Could you check a few things on this model? Use its own coordinates, in mm. A direction names the side the tool comes from. Give positions to 0.01 mm unless a question says otherwise; leave off trailing zeros. Loops run counter-clockwise (first coordinate to the right, second up) from the corner with the lowest first, then second, coordinate; pieces in that order, holes last. Notation, with made-up numbers: (36, 51.25) - (77, 51.25) arc R22 cw to (77, 57.25) - close; hole circle Ø2 at (58.5, 76). An arc over 180 degrees is marked (long way). Use CSV: the item, a comma, the result in double quotes.
from build123d import *

# Parameters (mm, degrees)
BOSS_EXTRUDE1_DEPTH       = 2
BOSS_EXTRUDE2_DEPTH       = 21.5
FILLET1_R                 = 2
FILLET2_R                 = 2
BOSS_EXTRUDE3_START       = -22
BOSS_EXTRUDE3_OUTLINE_R   = 1.498302823
BOSS_EXTRUDE3_OUTLINE_R_2 = 1.5
BOSS_EXTRUDE3_DEPTH       = 22
FILLET3_R                 = 2


with BuildPart() as part:
    # Sketch3 → Boss-Extrude1 (new body)
    with BuildSketch(Plane.XY):
        Polygon((-15.640963985, -84.058941087), (4.526340861, -63.891636241), (4.526340861, -11.788708514), (100.581340861, -11.788708514), (100.581340861, -63.896636241), (120.743645706, -84.058941087), (120.743645706, -106.958318205), (104.551340861, -106.958318205), (-15.640963985, -106.958318205), (-15.640963985, -90.76601336), align=None)
    extrude(amount=-BOSS_EXTRUDE1_DEPTH)

    # Sketch3<3> → Boss-Extrude2 (add)
    with BuildSketch(Plane.XY):
        Polygon((-15.640963985, -90.76601336), (-15.640963985, -84.058941087), (4.526340861, -63.891636241), (4.526340861, -11.788708514), (100.581340861, -11.788708514), (100.581340861, -63.896636241), (120.743645706, -84.058941087), (120.743645706, -106.958318205), (104.551340861, -106.958318205), (-15.640963985, -106.958318205), align=None)
        Polygon((-13.840963985, -90.76601336), (-13.840963985, -105.158318205), (104.551340861, -105.158318205), (118.943645706, -105.158318205), (118.943645706, -84.804525499), (98.781340861, -64.642220653), (98.781340861, -13.588708514), (6.326340861, -13.588708514), (6.326340861, -64.637220653), (-13.840963985, -84.804525499), align=None, mode=Mode.SUBTRACT)
    extrude(amount=BOSS_EXTRUDE2_DEPTH)

    # Fillet1
    fillet1_edges = [part.edges().sort_by_distance(p)[0] for p in [
        (-15.640963985, -84.058941087, 9.75),
        (4.526340861, -63.891636241, 9.75),
        (4.526340861, -11.788708514, 9.75),
        (100.581340861, -11.788708514, 9.75),
        (100.581340861, -63.896636241, 9.75),
        (120.743645706, -84.058941087, 9.75),
        (120.743645706, -106.958318205, 9.75),
        (-15.640963985, -106.958318205, 9.75),
        (-13.840963985, -105.158318205, 10.75),
        (-13.840963985, -84.804525499, 10.75),
        (6.326340861, -64.637220653, 10.75),
        (6.326340861, -13.588708514, 10.75),
        (98.781340861, -13.588708514, 10.75),
        (98.781340861, -64.642220653, 10.75),
        (118.943645706, -105.158318205, 10.75),
    ]]
    fillet(fillet1_edges, radius=FILLET1_R)

    # Fillet2
    fillet2_edges = [part.edges().sort_by_distance(p)[0] for p in [
        (118.943645706, -84.804525499, 10.75),
    ]]
    fillet(fillet2_edges, radius=FILLET2_R)

    # Boss-Extrude3: read off the stored shape, not the designer's step
    # Boss-Extrude3 outline → Boss-Extrude3 (add)
    with BuildSketch(Plane.XY.offset(21.5).offset(BOSS_EXTRUDE3_START)):
        with BuildLine():
            ThreePointArc((101.167127298, -64.482422679), (100.733581796, -63.833575981), (100.581340861, -63.068209116))
            Line((100.581340861, -63.068209116), (100.581340861, -13.788708514))
            ThreePointArc((100.581340861, -13.788708514), (99.995554423, -12.374494952), (98.581340861, -11.788708514))
            Line((98.581340861, -11.788708514), (6.526340861, -11.788708514))
            ThreePointArc((6.526340861, -11.788708514), (5.112127298, -12.374494952), (4.526340861, -13.788708514))
            Line((4.526340861, -13.788708514), (4.526340861, -63.063209116))
            ThreePointArc((4.526340861, -63.063209116), (4.374099926, -63.828575981), (3.940554423, -64.477422679))
            Line((3.940554423, -64.477422679), (-15.055177547, -83.473154649))
            ThreePointArc((-15.055177547, -83.473154649), (-15.48872305, -84.122001347), (-15.640963985, -84.887368211))
            Line((-15.640963985, -84.887368211), (-15.640963985, -104.958318205))
            ThreePointArc((-15.640963985, -104.958318205), (-15.055177547, -106.372531767), (-13.640963985, -106.958318205))
            Line((-13.640963985, -106.958318205), (118.743645706, -106.958318205))
            ThreePointArc((118.743645706, -106.958318205), (120.157859269, -106.372531767), (120.743645706, -104.958318205))
            Line((120.743645706, -104.958318205), (120.743645706, -84.887368211))
            ThreePointArc((120.743645706, -84.887368211), (120.591404771, -84.122001347), (120.157859269, -83.473154649))
            Line((120.157859269, -83.473154649), (101.167127298, -64.482422679))
        make_face()
        with Locations((-12.195717461, -103.513071681)):
            Circle(BOSS_EXTRUDE3_OUTLINE_R, mode=Mode.SUBTRACT)
        with Locations((-1.913886606, -74.998768464)):
            Circle(BOSS_EXTRUDE3_OUTLINE_R_2, mode=Mode.SUBTRACT)
        with Locations((52.551340861, -103.658318205)):
            Circle(BOSS_EXTRUDE3_OUTLINE_R_2, mode=Mode.SUBTRACT)
        with Locations((117.297199097, -103.511871596)):
            Circle(BOSS_EXTRUDE3_OUTLINE_R_2, mode=Mode.SUBTRACT)
        with Locations((107.016568327, -74.998768464)):
            Circle(BOSS_EXTRUDE3_OUTLINE_R_2, mode=Mode.SUBTRACT)
        with BuildLine():
            ThreePointArc((-13.840963985, -85.632952624), (-13.68872305, -84.867585759), (-13.255177547, -84.218739061))
            Line((-13.255177547, -84.218739061), (-4.688095726, -75.651657241))
            ThreePointArc((-4.688095726, -75.651657241), (0.101367721, -77.01402279), (-1.260997829, -72.224559343))
            Line((-1.260997829, -72.224559343), (5.740554423, -65.223007091))
            ThreePointArc((5.740554423, -65.223007091), (6.174099926, -64.574160393), (6.326340861, -63.808793529))
            Line((6.326340861, -63.808793529), (6.326340861, -17.561464123))
            ThreePointArc((6.326340861, -17.561464123), (9.988041797, -17.25040945), (10.29909647, -13.588708514))
            Line((10.29909647, -13.588708514), (50.130516698, -13.588708514))
            ThreePointArc((50.130516698, -13.588708514), (52.553840861, -17.938708514), (54.977165024, -13.588708514))
            Line((54.977165024, -13.588708514), (94.808585252, -13.588708514))
            ThreePointArc((94.808585252, -13.588708514), (95.119639925, -17.25040945), (98.781340861, -17.561464123))
            Line((98.781340861, -17.561464123), (98.781340861, -63.813793529))
            ThreePointArc((98.781340861, -63.813793529), (98.933581796, -64.579160393), (99.367127298, -65.228007091))
            Line((99.367127298, -65.228007091), (106.36367955, -72.224559343))
            ThreePointArc((106.36367955, -72.224559343), (105.001314001, -77.01402279), (109.790777448, -75.651657241))
            Line((109.790777448, -75.651657241), (118.357859269, -84.218739061))
            ThreePointArc((118.357859269, -84.218739061), (118.791404771, -84.867585759), (118.943645706, -85.632952624))
            Line((118.943645706, -85.632952624), (118.943645706, -101.185562596))
            ThreePointArc((118.943645706, -101.185562596), (115.28194477, -101.496617269), (114.970890097, -105.158318205))
            Line((114.970890097, -105.158318205), (54.974665024, -105.158318205))
            ThreePointArc((54.974665024, -105.158318205), (52.551340861, -100.808318205), (50.128016698, -105.158318205))
            Line((50.128016698, -105.158318205), (-9.870638356, -105.158318205))
            ThreePointArc((-9.870638356, -105.158318205), (-10.18166322, -101.49901744), (-13.840963985, -101.187992576))
            Line((-13.840963985, -101.187992576), (-13.840963985, -85.632952624))
        make_face(mode=Mode.SUBTRACT)
        with Locations((7.97278747, -15.235155124)):
            Circle(BOSS_EXTRUDE3_OUTLINE_R_2, mode=Mode.SUBTRACT)
        with Locations((52.553840861, -15.088708514)):
            Circle(BOSS_EXTRUDE3_OUTLINE_R_2, mode=Mode.SUBTRACT)
        with Locations((97.134894251, -15.235155124)):
            Circle(BOSS_EXTRUDE3_OUTLINE_R_2, mode=Mode.SUBTRACT)
    extrude(amount=BOSS_EXTRUDE3_DEPTH)

    # Fillet3
    fillet3_edges = [part.edges().sort_by_distance(p)[0] for p in [
        (10.29909647, -13.588708514, 10.75),
        (6.326340861, -17.561464123, 10.75),
        (54.977165024, -13.588708514, 10.75),
        (50.130516698, -13.588708514, 10.75),
        (94.808585252, -13.588708514, 10.75),
        (98.781340861, -17.561464123, 10.75),
        (109.790777448, -75.651657241, 10.75),
        (106.36367955, -72.224559343, 10.75),
        (118.943645706, -101.185562596, 10.75),
        (114.970890097, -105.158318205, 10.75),
        (50.128016698, -105.158318205, 10.75),
        (54.974665024, -105.158318205, 10.75),
        (-9.870638356, -105.158318205, 10.75),
        (-13.840963985, -101.187992576, 10.75),
        (-4.688095726, -75.651657241, 10.75),
        (-1.260997829, -72.224559343, 10.75),
    ]]
    fillet(fillet3_edges, radius=FILLET3_R)


solid = part.part
1) Suppose I cut it at B-B (y = -87.5). Please give me the cut outline in (x, z).
Answer below:
outline,"(-15.64, -2) - (120.74, -2) - (120.74, 21.5) - (118.94, 21.5) - (118.94, 0) - (-13.84, 0) - (-13.84, 21.5) - (-15.64, 21.5) - close"
2) We'd pull the mould along Y, two halves only. Please class faces 4 (the flat face through (-15.641, -95, 10)), 5 (the flat face through (-5.69, -74.11, 9.59)), 6 (the flat face through (102.05, -67.91, 10.6)): +Y half, -Y half, draft (parallel to the pull), parting line (faces both ways), or undercut.
Answer below:
face 4,"draft"
face 5,"+Y half"
face 6,"undercut"
3) Suppose I cut it at C-C (z = 2). State how many separate pieces and enclosed holes the cut face has, plus the area to 3 significant figures.
Answer below:
separate pieces,"1"
enclosed holes,"9"
area,"890 mm2"
4) I'm going to push flat-ended pins straight in: P1, Ø1, axis at y = -55, z = 9, coming from the -X side; P2, Ø0.9, axis at x = 106.5, y = -74.5, coming from the +Z side; P3, Ø10, axis at y = -69, z = 7, coming from the -X side. Where does each tip first touch, or does it pass through?
Answer below:
P1,"stops at x = 4.53"
P2,"stops at z = 0"
P3,"stops at x = -5.58"
5) I need wall thicknesses on line 1 along X through (y, z) = (-26.5, 12); line 2 along Y through (x, z) = (25.5, 14.5); line 3 along X through (y, z) = (-77.5, 3.5). Which ranges of each line are inside material? Lowest first, please.
Answer below:
line 1,"x = 4.53 to 6.33, 98.78 to 100.58"
line 2,"y = -106.96 to -105.16, -13.59 to -11.79"
line 3,"x = -9.08 to -6.54, -3.28 to -0.55, 105.65 to 108.38, 111.64 to 114.18"
6) Which directions (+Z, -Z, +X, -X, +Y, -Y) give clear straight access to the entire face, cutting with the end or side of a thin tool? Please do faces 1 (the flat face through (53, -17, 21.5)), 2 (the cylindrical face through (9.97, -17.27, 10.6)), 3 (the flat face through (100.581, -38, 10)).
Answer below:
face 1,"+Z, +X, -X, +Y, -Y"
face 2,"+Z"
face 3,"+Z, -Z, +X, +Y"
7) Suppose I cut it at A-A (x = 17.5). Please give me the cut outline in (y, z).
Answer below:
outline,"(-106.96, -2) - (-11.79, -2) - (-11.79, 21.5) - (-13.59, 21.5) - (-13.59, 0) - (-105.16, 0) - (-105.16, 21.5) - (-106.96, 21.5) - close"
